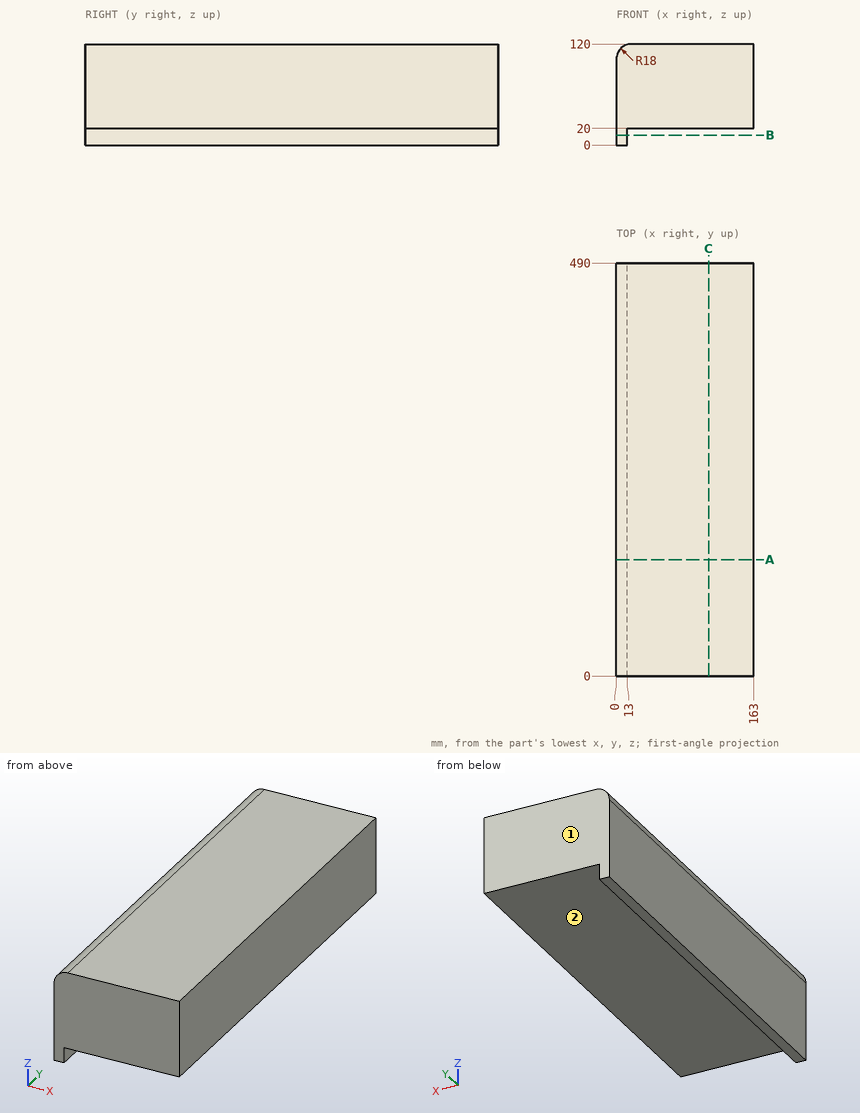
Geometry check sheet. Reference: drawing and pictorial views, mm from the part's lowest x, y, z. A direction names the side the tool comes from. Give positions to 0.01 mm unless a question says otherwise; leave off trailing zeros. Order: outer loops, then holes, each group sorted by start corner. A loop starts at its lowest first (then second) coordinate and runs counter-clockwise, first axis right, second up. Notation, with made-up numbers: (1.25, 72.25) -> (19.25, 72.25) arc R19 cw to (19.25, 98.25) -> close; hole circle Ø7 at (62, 67.5). An arc over 180 degrees is marked (long way). Write each question's results on one line, items separated by ' | '. Start each with the question number.
(1) Sectioned sample at C-C (x = 109.5). Enter the section's corners in (y, z).
(2) Scan lines: line 1 (Z direction, x = 87, y = 25); line 2 (X direction, y = 442, z = 11.5); line 3 (X direction, y = 154.5, z = 112.5). Record each from-to range of solid material in increasing order.
(3) Access from +Z, -Z, +X, -X, +Y, -Y to the whole of each face (thin tool, end or side, straight path). Record for the marked faces 1 and 2.
(4) Sectioned sample at A-A (y = 138). Enter the section's corners in (x, z).
(5) Gauge pin test, flat ends, axial feed: P1, Ø12, axis at x = 105, z = 48.5, coming from the -Y side; P2, Ø22, axis at y = 187.5, z = 7.5, coming from the +X side; P3, Ø1.5, axis at x = 44.5, y = 322.5, coming from the -Z side. Record the tip position at first contact, or that the pin passes through.
(6) Sectioned sample at B-B (z = 12). Enter the section's corners in (x, y), plus the area to 3 significant figures.
Answer below:
1) outline: (0, 20) -> (490, 20) -> (490, 120) -> (0, 120) -> close
2) line 1: 20 to 120 | line 2: 0 to 13 | line 3: 3.38 to 163
3) face 1: +Z, -Z, +X, -X, +Y | face 2: -Z, +X, +Y, -Y
4) outline: (0, 0) -> (13, 0) -> (13, 20) -> (163, 20) -> (163, 120) -> (18, 120) arc R18 ccw to (0, 102) -> close
5) P1: y = 0 | P2: x = 13 | P3: z = 20
6) outline: (0, 0) -> (13, 0) -> (13, 490) -> (0, 490) -> close | area: 6,370 mm2
